Check sheet for the modelled part. Datum: model origin and axes. Units: mm. A direction names the side the tool comes from. Round coordinates to 2 decimals unless told otherwise and drop trailing zeros. Order: outer loops, then holes, each group sorted by start corner. A loop starts at its lowest first (then second) coordinate and runs counter-clockwise, first axis right, second up.
```python
from build123d import *

# Parameters (mm, degrees)
F1_DEPTH = 6.35
F2_R     = 4.22275
F3_DEPTH = 6.351
F4_R     = 2.54


# Not quite as in the source:
# - a length typed as a fraction of an inch, garbled in the dataset ("3 / 203.2 mm" for 3/8 in), is restored


with BuildPart() as f1:
    # F0 (on Top) → F1 (new body)
    with BuildSketch(Plane.XY):
        Polygon((0, 78.937935479), (-38.1, 78.937935479), (-38.1, -22.662064521), (63.5, -22.662064521), (63.5, 15.437935479), (0, 15.437935479), align=None)
    extrude(amount=F1_DEPTH)

    # F2 (on face) → F3 (cut, through all)
    with BuildSketch(Plane.XY.offset(6.35)):
        with Locations((-27.52725, 68.365185479)):
            Circle(F2_R)
        with Locations((-10.57275, 68.365185479)):
            Circle(F2_R)
        with Locations((52.92725, 4.865185479)):
            Circle(F2_R)
        with Locations((52.92725, -12.089314521)):
            Circle(F2_R)
        with Locations((-27.52725, -12.089314521)):
            Circle(F2_R)
    extrude(amount=-F3_DEPTH, mode=Mode.SUBTRACT)

    # F4
    f4_edges = [f1.edges().sort_by_distance(p)[0] for p in [
        (-38.1, -22.662065, 3.175),
        (63.5, -22.662065, 3.175),
        (63.5, 15.437935, 3.175),
        (0, 15.437935, 3.175),
        (0, 78.937935, 3.175),
        (-38.1, 78.937935, 3.175),
    ]]
    fillet(f4_edges, radius=F4_R)


solid = f1.part
```
Item 1: Access from +Z, -Z, +X, -X, +Y, -Y to the whole of each face (thin tool, end or side, straight path). Record for faces 4 (the flat face through (0, 47, 3)), 5 (the cylindrical face through (-8.62, 64.62, 3.22)).
Answer:
face 4: +Z, -Z, +X, +Y
face 5: +Z, -Z
Item 2: Sectioned sample at C-C (z = 4). Record the cut outline in (x, y), and give its area (3 significant figures).
Answer:
outline: (-38.1, -20.12) arc R2.54 ccw to (-35.56, -22.66) - (60.96, -22.66) arc R2.54 ccw to (63.5, -20.12) - (63.5, 12.9) arc R2.54 ccw to (60.96, 15.44) - (2.54, 15.44) arc R2.54 cw to (0, 17.98) - (0, 76.4) arc R2.54 ccw to (-2.54, 78.94) - (-35.56, 78.94) arc R2.54 ccw to (-38.1, 76.4) - close; hole circle Ø8.45 at (-27.53, -12.09); hole circle Ø8.45 at (-27.53, 68.37); hole circle Ø8.45 at (-10.57, 68.37); hole circle Ø8.45 at (52.93, -12.09); hole circle Ø8.45 at (52.93, 4.87)
area: 6,000 mm2
Item 3: Sectioned sample at D-D (x = -29). Record the cut outline in (y, z).
Answer:
outline: (-22.66, 0) - (-16.05, 0) - (-16.05, 6.35) - (-22.66, 6.35) - close; (-8.13, 0) - (64.41, 0) - (64.41, 6.35) - (-8.13, 6.35) - close; (72.32, 0) - (78.94, 0) - (78.94, 6.35) - (72.32, 6.35) - close
Item 4: Scan lines: line 1 along Y through (x, z) = (52.5, 5); line 2 along Y through (x, z) = (55.5, 2.5); line 3 along X through (y, z) = (-14, 5.25). Record each from-to range of solid material in increasing order.
Answer:
line 1: y = -22.66 to -16.29, -7.89 to 0.66, 9.07 to 15.44
line 2: y = -22.66 to -15.44, -8.74 to 1.52, 8.21 to 15.44
line 3: x = -38.1 to -31.29, -23.76 to 49.16, 56.69 to 63.5
Item 5: Release check for a two-part mould opening along Y. For faces 1 (the cylindrical face through (56.83, 3.25, 3.22)), 2 (the cylindrical face through (62.74, 14.71, 3.22)), 3 (the flat face through (63.5, -4, 3)) record: released by +Y, released by -Y, zero draft, split by the parting line, or undercut.
Answer:
face 1: undercut
face 2: released by +Y
face 3: zero draft
Item 6: Go/stop test with flat-tipped pins: P1, Ø13.5, axis at x = -27.53, y = 68.37, coming from the -Z side; P2, Ø3, axis at x = 22, z = 4, coming from the +Y side. Record where each tip stops, or that it passes through.
Answer:
P1: stops at z = 0
P2: stops at y = 15.44
Item 7: Sectioned sample at B-B (y = -9.5). Record the cut outline in (x, z).
Answer:
outline: (-38.1, 0) - (-30.86, 0) - (-30.86, 6.35) - (-38.1, 6.35) - close; (-24.19, 0) - (49.59, 0) - (49.59, 6.35) - (-24.19, 6.35) - close; (56.26, 0) - (63.5, 0) - (63.5, 6.35) - (56.26, 6.35) - close
Item 8: Sectioned sample at A-A (x = -9.5). Record the cut outline in (y, z).
Answer:
outline: (-22.66, 0) - (64.28, 0) - (64.28, 6.35) - (-22.66, 6.35) - close; (72.45, 0) - (78.94, 0) - (78.94, 6.35) - (72.45, 6.35) - close
